Geometry: final body of the model. Coordinates: model frame, mm. Coordinates: 2 decimals unless noted, no trailing zeros. Write each loop counter-clockwise with the first axis right and the second up, starting at its lowest first coordinate (ties: lowest second). Pieces come first, ordered by that corner, then holes. Notation, with made-up numbers: (60.25, -12.75) - (71.25, -12.75) arc R10 cw to (71.25, -4.75) - close; hole circle Ø9 at (-13, -20). An arc over 180 degrees is marked (long way). Put each result on its own line as item: value.
```python
from build123d import *

# Parameters (mm, degrees)
SKETCH_1_R          = 15
EXTRUDE_1_DEPTH     = 4
HOLE_WIZARD_M3_1_D  = 3.4
FILLET_7_R          = 7.5
FILLET_8_R          = 3.5
SKETCH_4_W          = 12
SKETCH_4_H          = 118
CUT_EXTRUDE_1_DEPTH = 221.649609109
FILLET_9_R          = 3


with BuildPart() as part:
    # ｽｹｯﾁ1 → ﾎﾞｽ - 押し出し1 (new body)
    with BuildSketch(Plane(origin=(0, 0, 0), x_dir=(0, 1, 0), z_dir=(0, 0, 1))):
        Polygon((0, 0), (148, 0), (148, 45), (170.5, 45), (170.5, 95), (148, 95), (148, 140), (0, 140), (0, 95), (-22.5, 95), (-22.5, 45), (0, 45), align=None)
        with Locations(Location((2.5, 70, 0), (0, 0, 270))):
            Circle(SKETCH_1_R, mode=Mode.SUBTRACT)
        with Locations(Location((145.5, 70, 0), (0, 0, 90))):
            Circle(SKETCH_1_R, mode=Mode.SUBTRACT)
    extrude(amount=EXTRUDE_1_DEPTH)

    # M3 すきま穴1 (through all)
    with Locations(Plane.XY.offset(4)):
        with Locations((-132.5, 140.5), (-7.5, 140.5), (-106.2, 51.02), (-30, 98.01), (-7.5, 7.5), (-132.5, 7.5), (-82.07, 64.99), (-136, 107.3), (-89.4, 107.3), (-89.4, 40.7), (-136, 40.7), (-91.5, 24), (-48.5, 24), (-48.5, -19), (-91.5, -19), (-91.5, 167), (-48.5, 167), (-48.5, 124), (-91.5, 124)):
            Hole(HOLE_WIZARD_M3_1_D / 2)

    # ﾌｨﾚｯﾄ7
    fillet_7_edges = [part.edges().sort_by_distance(p)[0] for p in [
        (-45, 0, 2),
        (-95, 0, 2),
        (-140, 0, 2),
        (-140, 148, 2),
        (-95, 148, 2),
        (-45, 148, 2),
        (0, 148, 2),
        (0, 0, 2),
    ]]
    fillet(fillet_7_edges, radius=FILLET_7_R)

    # ﾌｨﾚｯﾄ8
    fillet_8_edges = [part.edges().sort_by_distance(p)[0] for p in [
        (-45, -22.5, 2),
        (-95, -22.5, 2),
        (-95, 170.5, 2),
        (-45, 170.5, 2),
    ]]
    fillet(fillet_8_edges, radius=FILLET_8_R)

    # ｽｹｯﾁ4 → ｶｯﾄ - 押し出し1 (cut, through all)
    with BuildSketch(Plane.XY.offset(4)):
        with Locations((-122, 74)):
            Rectangle(SKETCH_4_W, SKETCH_4_H)
        with BuildLine():
            Line((-64, 145.5), (-64, 2.5))
            ThreePointArc((-64, 2.5), (-70, -3.5), (-76, 2.5))
            Line((-76, 2.5), (-76, 145.5))
            ThreePointArc((-76, 145.5), (-70, 151.5), (-64, 145.5))
        make_face()
        with Locations((-18, 74)):
            Rectangle(SKETCH_4_W, SKETCH_4_H)
    extrude(amount=-CUT_EXTRUDE_1_DEPTH, mode=Mode.SUBTRACT)

    # ﾌｨﾚｯﾄ9
    fillet_9_edges = [part.edges().sort_by_distance(p)[0] for p in [
        (-76, 131.752272915, 2),
        (-64, 131.752272915, 2),
        (-128, 15, 2),
        (-128, 133, 2),
        (-116, 133, 2),
        (-116, 15, 2),
        (-64, 16.247727085, 2),
        (-76, 16.247727085, 2),
        (-12, 133, 2),
        (-12, 15, 2),
        (-24, 15, 2),
        (-24, 133, 2),
    ]]
    fillet(fillet_9_edges, radius=FILLET_9_R)


solid = part.part
```
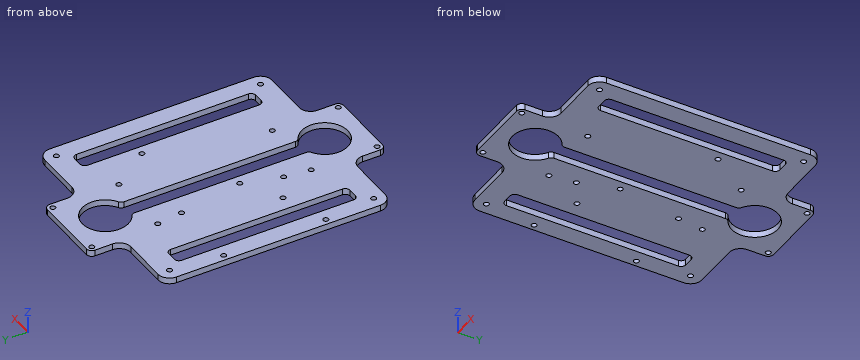
1. Section query C-C (z = 2.05). Count the separate pieces of the cut face and the enclosed holes in it, then the cut area to 3 significant figures.
Answer below:
separate pieces: 1
enclosed holes: 22
area: 17,200 mm²
2. Section query B-B (x = -58.5). Return loops of the section in (y, z), then the cut area to 3 significant figures.
Answer below:
outline: (-22.5, 0) - (-7.13, 0) - (-7.13, 4) - (-22.5, 4) - close; (12.13, 0) - (135.87, 0) - (135.87, 4) - (12.13, 4) - close; (155.13, 0) - (170.5, 0) - (170.5, 4) - (155.13, 4) - close
area: 618 mm²
3. Ray query, probe 1 along X at (y, z) = (107, 2.55); probe 2 along Y at (x, z) = (-91.5, 2.5); probe 3 along Y at (x, z) = (-132.5, 2.05). Return the intervals inside material, ascending. Write a range as from..to.
Answer below:
probe 1: x = -140..-137.67, -134.33..-128, -116..-91.07, -87.73..-76, -64..-24, -12..0
probe 2: y = -22.5..-20.7, -17.3..22.3, 25.7..122.3, 125.7..165.3, 168.7..170.5
probe 3: y = 0..5.8, 9.2..138.8, 142.2..148
4. Section query A-A (y = 113.5). Return loops of the section in (x, z), then the cut area to 3 significant figures.
Answer below:
outline: (-140, 0) - (-128, 0) - (-128, 4) - (-140, 4) - close; (-116, 0) - (-76, 0) - (-76, 4) - (-116, 4) - close; (-64, 0) - (-24, 0) - (-24, 4) - (-64, 4) - close; (-12, 0) - (0, 0) - (0, 4) - (-12, 4) - close
area: 416 mm²
5. Pin query (flat end, axial travel): pin 1 Ø3 at (x, y) = (-7.5, 7.5) entering from -Z; pin 2 Ø1.2 at (x, z) = (-122.5, 1) entering from +Y; pin 3 Ø2 at (x, z) = (-19, 1.5) entering from -Y. Return the tip coordinate at first contact, or that it passes through.
Answer below:
pin 1: passes through
pin 2: stops at y = 148
pin 3: stops at y = 0
